```python
from build123d import *

# Parameters (mm, degrees)
F0_W     = 127
F0_H     = 127
F1_DEPTH = 2.54
F3_D     = 20.32


with BuildPart() as f1:
    # F0 (on Top) → F1 (new body)
    with BuildSketch(Plane.XY):
        with Locations((21.668797, 23.006538)):
            Rectangle(F0_W, F0_H)
    extrude(amount=F1_DEPTH)

    # F3 (through all)
    with Locations(Plane.XY.offset(2.54)):
        with Locations((21.668797, 23.006538)):
            Hole(F3_D / 2)


solid = f1.part
```
Can you work these out from the model? Positions are in its coordinate system, mm. Give positions to 0.01 mm unless a question says otherwise; leave off trailing zeros. Loops run counter-clockwise (first coordinate to the right, second up) from the corner with the lowest first, then second, coordinate; pieces in that order, holes last. Notation, with made-up numbers: M 50,57.25 L 105,57.25 A36 cw 105,92.25 Z; hole C 52,54 d2. An arc over 180 degrees is marked long. Answer in a Markdown table with one row per item.
1. Suppose I cut it at A-A on y = 29. Write out the boundary of the cut face in (x, z), plus the area to 3 significant figures.
Taken from the geometry:
| item | result |
|---|---|
| outline | M -41.83,0 L 13.46,0 L 13.46,2.54 L -41.83,2.54 Z; M 29.87,0 L 85.17,0 L 85.17,2.54 L 29.87,2.54 Z |
| area | 281 mm² |
2. If I drill on line 1 along Y through (x, z) = (28, 1.55); line 2 along X through (y, z) = (22, 1.2), over which ranges is the centre line in solid material (lowest first)?
Taken from the geometry:
| item | result |
|---|---|
| line 1 | y = -40.49 to 15.06, 30.95 to 86.51 |
| line 2 | x = -41.83 to 11.56, 31.78 to 85.17 |
3. Thinking about a two-plate mould opening in Y: for faces 1 (the flat face through (35, 24, 2.54)), 2 (the cylindrical face through (22.99, 33.08, 1.25)), which applies, released by +Y, released by -Y, zero draft, split by the parting line, or undercut?
Taken from the geometry:
| item | result |
|---|---|
| face 1 | zero draft |
| face 2 | undercut |
4. For pin 1 Ø18.5 at (x, y) = (21.67, 23.01) entering from +Z, with a flat end and sliding along its axis, tell me the tip position at first contact or that it passes through.
Taken from the geometry:
| item | result |
|---|---|
| pin 1 | passes through |
5. Suppose I cut it at B-B on z = 2.15. Write out the boundary of the cut face in (x, y), plus the area to 3 significant figures.
Taken from the geometry:
| item | result |
|---|---|
| outline | M -41.83,-40.49 L 85.17,-40.49 L 85.17,86.51 L -41.83,86.51 Z; hole C 21.67,23.01 d20.32 |
| area | 15,800 mm² |
